The listing builds one solid part. Answer for the finished solid, in the listing's coordinates (mm). A direction names the side the tool comes from. Coordinates: 2 decimals unless noted, no trailing zeros. Write each loop counter-clockwise with the first axis right and the second up, starting at its lowest first coordinate (ties: lowest second). Pieces come first, ordered by that corner, then holes. Notation, with made-up numbers: M 29,66 L 42,66 A15 cw 42,90 Z; hole C -35,-4.75 d5. An arc over 180 degrees is marked long. Answer as a JSON object with one key per item and string values. Group by question number.
Autodesk Inventor part; units mm, degrees
ref_plane "YZ Plane" through (0, 0, 0) normal (1, 0, 0) x (0, 1, 0)
ref_plane "XZ Plane" through (0, 0, 0) normal (0, 1, 0) x (-1, 0, 0)
ref_plane "XY Plane" through (0, 0, 0) normal (0, 0, 1) x (1, 0, 0)
sketch "Boceto10" plane through (0, 0, 0) normal (0, 0, 1) x (1, 0, 0)
  line L0 (93.7879, -1.2643) -> (379.7634, -26.5882)
  line L1 (93.7879, -1.2643) -> (118.6905, -3.4695)
  line L2 (118.6905, -3.4695) -> (115.1622, -43.3135)
  line L3 (115.1622, -43.3135) -> (155.0063, -46.8418)
  line L4 (155.0063, -46.8418) -> (158.5346, -6.9978)
  line L5 (158.5346, -6.9978) -> (118.6905, -3.4695)
  line L6 (156.366, -8.8135) -> (153.1905, -44.6732)
  line L7 (153.1905, -44.6732) -> (117.3308, -41.4977)
  line L8 (117.3308, -41.4977) -> (120.5063, -5.6381)
  line L9 (120.5063, -5.6381) -> (156.366, -8.8135)
  line L10 (118.6905, -3.4695) -> (115.1622, -43.3135)
  line L11 (115.1622, -43.3135) -> (155.0063, -46.8418)
  line L12 (155.0063, -46.8418) -> (158.5346, -6.9978)
  line L13 (158.5346, -6.9978) -> (118.6905, -3.4695)
  point P0 (0, 0)
  dimension "d40" = 25
  dimension "l_c" = 40
  dimension "l_c2" = 40
  dimension "l_c3" = 40
  dimension "t_c" = 2
extrude "Extrusión2" add sketch "Boceto10" against normal blind 900
sketch "Boceto12" plane through (158.5346, -6.9978, 0) normal (0.0882, 0.9961, 0) x (0.9961, -0.0882, 0)
  line L0 (-20, -27) -> (-20, 93.85)
  circle A0 centre (-20, 93.85) radius 4
  line L1 (-38, 900) -> (-2, 900)
  line L2 (-20, 900) -> (-20, 806.15)
  circle A1 centre (-20, 806.15) radius 4
  line L3 (-20, 93.85) -> (-20, 806.15)
  line L4 (0, 0) -> (-40, 0)
  line L5 (-40, 0) -> (-40, 108)
  line L6 (-40, 0) -> (-40, 900)
  point P0 (-158.5339, 0)
  dimension "d49" = 8
  dimension "d51" = 8
  dimension "d59" = 712.3
  dimension "d60" = 93.85
  dimension "d61" = 108
hole "Agujero1" at (138.6125, -5.2336, -93.85) at (138.6125, -5.2336, -806.15) direction (-0.0882, -0.9961, 0) diameter 8 end through all
equation "\"l_c2\" = l_c"
equation "\"l_c3\" = l_c"
properties part number "Asiento nuevo" material "Acero, suave"
Item 1: A cutting plane is placed at B-B, the plane y = -22. Write down the section's boundary in (x, z), and give its area (3 significant figures).
Item 2: Flat-ended cylindrical pins translate along their axes: pin 1 Ø10 at (y, z) = (-20, -395.5) entering from +X; pin 2 Ø5 at (x, y) = (121.5, -15.5) entering from -Z; pin 3 Ø4 at (y, z) = (-18, -362) entering from -X; pin 4 Ø10 at (x, y) = (135.5, -36.5) entering from -Z. Find the tip coordinate at first contact, or state that the pin passes through.
Item 3: Consider L1, parallel to Z at x = 133.5, y = -43.5; L2, parallel to X at y = -26, z = -756; L3, parallel to Y at x = 141.5, z = -688.5. Determine where each line is inside the solid, lowest interval first. Write a range as from..to.
Item 4: For a pull along X with two mould halves and no side action, classify faces 1 (the face through (138.185, -7.204, -443.7)), 2 (the face through (138.33, -5.21, -443.7)), 3 (the face through (130, -43, 0)) as +X half, -X half, draft (parallel to the pull), parting line (faces both ways), or undercut.
Item 5: A tool of negligible diameter and unlimited length cuts with its end or side. For faces 4 (the face through (154.8, -26.5, -443.7)), 5 (the face through (116.95, -23.11, -443.7)), from which of +Z, -Z, +X, -X, +Y, -Y can it reach the whole face along a straight path? Write none if from no direction.
Item 6: A cutting plane is placed at A-A, the plane z = -733. Write down the section's boundary in (x, y).
Answer:
{
 "1": {"outline": "M 117.05,-900 L 119.06,-900 L 119.06,0 L 117.05,0 Z; M 155.2,-900 L 157.21,-900 L 157.21,0 L 155.2,0 Z", "area": "3,610 mm2"},
 "2": {"pin 1": "x = 157.83", "pin 2": "z = -900", "pin 3": "x = 117.23", "pin 4": "through"},
 "3": {"L1": "-900..-809.76, -802.54..-97.46, -90.24..0", "L2": "116.7..118.7, 154.84..156.85", "L3": "-45.65..-43.64, -7.5..-5.49"},
 "4": {"face 1": "undercut", "face 2": "+X half", "face 3": "draft"},
 "5": {"face 4": "+Z, -Z", "face 5": "+Z, -Z, -X, +Y"},
 "6": {"outline": "M 115.16,-43.31 L 155.01,-46.84 L 158.53,-7 L 118.69,-3.47 Z; hole M 117.33,-41.5 L 153.19,-44.67 L 156.37,-8.81 L 120.51,-5.64 Z"}
}
